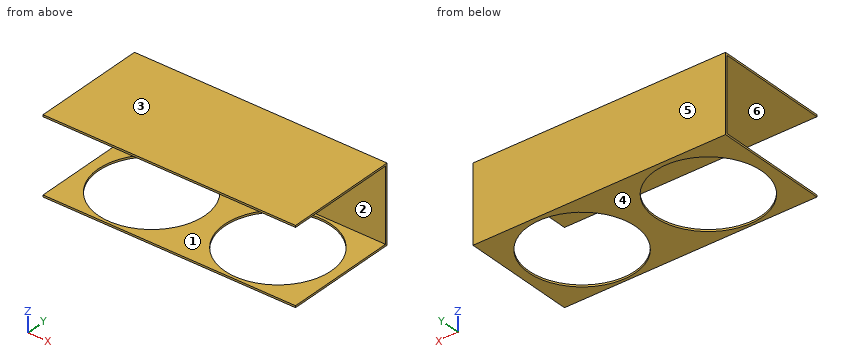
```python
from build123d import *

# Parameters (mm, degrees)
F0_W          = 270
F0_H          = 2
F0_H_2        = 120
F0_R          = 57
F1_DEPTH      = 2
F2_DEPTH      = 80
F3_W          = 270
F3_H          = 2
F4_DEPTH      = 120
F4_DEPTH_BACK = 2


with BuildPart() as f1:
    # F0 (on Top) → F1 (new body)
    with BuildSketch(Plane.XY):
        with Locations((13.665279, 62.509182)):
            Rectangle(F0_W, F0_H)
        with Locations((13.665279, 1.509182)):
            Rectangle(F0_W, F0_H_2)
        with Locations((-53.288383, 1.509182)):
            Circle(F0_R, mode=Mode.SUBTRACT)
        with Locations((81.711617, 1.509182)):
            Circle(F0_R, mode=Mode.SUBTRACT)
    extrude(amount=F1_DEPTH)

    # F0 (on Top) → F2 (join)
    with BuildSketch(Plane.XY):
        with Locations((13.665279, 62.509182)):
            Rectangle(F0_W, F0_H)
    extrude(amount=F2_DEPTH)

    # F3 (on face) → F4 (join, two sides)
    with BuildSketch(Plane.XZ.offset(-61.509182)) as f4_sk:
        with Locations((13.665279, 81)):
            Rectangle(F3_W, F3_H)
    extrude(amount=F4_DEPTH)
    extrude(f4_sk.sketch, amount=-F4_DEPTH_BACK)


solid = f1.part
```
Geometry check sheet. Reference: the model listing, model coordinates, mm. Face numbers are marked on the shaded views. A direction names the side the tool comes from. Coordinates: 2 decimals unless noted, no trailing zeros. Order: outer loops, then holes, each group sorted by start corner. A loop starts at its lowest first (then second) coordinate and runs counter-clockwise, first axis right, second up. Notation, with made-up numbers: (30, -32) - (59, -32) arc R20 ccw to (59, -6) - close; hole circle Ø1 at (6, -38.5). An arc over 180 degrees is marked (long way). Answer as a JSON object with one key per item and string values. Group by question number.
Item 1: Sectioned sample at B-B, the plane y = 22.5. Record the cut outline in (x, z), and give its area (3 significant figures).
Item 2: Sectioned sample at D-D, the plane z = 77. Record the cut outline in (x, y), and give its area (3 significant figures).
Item 3: Sectioned sample at C-C, the plane x = 13.5. Record the cut outline in (y, z), and give its area (3 significant figures).
Item 4: Tool access check on the marked faces 5 and 6. Record the directions out of +Z, -Z, +X, -X, +Y, -Y that give a thin tool (end or side, any length) a straight path to the whole face; none if there is none.
Item 5: Scan lines: probe 1 along Z at (x, y) = (20, -13); probe 2 along Y at (x, z) = (-15, 78); probe 3 along Z at (x, y) = (27, 5.5). Record each from-to range of solid material in increasing order.
Item 6: Depth check by flat-ended pin: pin 1 Ø1.5 at (x, y) = (-29, -27) entering from -Z; pin 2 Ø1 at (x, z) = (56, 50) entering from -Y. Enter the tip coordinate at first touch or a pass-through.
Item 7: Sectioned sample at A-A, the plane x = -37. Record the cut outline in (y, z).
Item 8: Draft check along Z on the marked faces 1, 2, 3 and 4. Enter one of: +Z half, -Z half, draft (parallel to the pull), parting line (faces both ways), or undercut.
Resolved:
{
 "1": {"outline": "(-121.33, 0) - (-106.28, 0) - (-106.28, 2) - (-121.33, 2) - close; (-121.33, 80) - (148.67, 80) - (148.67, 82) - (-121.33, 82) - close; (-0.29, 0) - (28.72, 0) - (28.72, 2) - (-0.29, 2) - close; (134.71, 0) - (148.67, 0) - (148.67, 2) - (134.71, 2) - close", "area": "656 mm^2"},
 "2": {"outline": "(-121.33, 61.51) - (148.67, 61.51) - (148.67, 63.51) - (-121.33, 63.51) - close", "area": "540 mm^2"},
 "3": {"outline": "(-58.49, 0) - (63.51, 0) - (63.51, 82) - (-58.49, 82) - (-58.49, 80) - (61.51, 80) - (61.51, 2) - (-58.49, 2) - close", "area": "644 mm^2"},
 "4": {"face 5": "+Z, -Z, +X, -X, +Y", "face 6": "+X, -X, -Y"},
 "5": {"probe 1": "0 to 2, 80 to 82", "probe 2": "61.51 to 63.51", "probe 3": "80 to 82"},
 "6": {"pin 1": "z = 80", "pin 2": "y = 61.51"},
 "7": {"outline": "(-58.49, 0) - (-53.11, 0) - (-53.11, 2) - (-58.49, 2) - close; (-58.49, 80) - (61.51, 80) - (61.51, 2) - (56.13, 2) - (56.13, 0) - (63.51, 0) - (63.51, 82) - (-58.49, 82) - close"},
 "8": {"face 1": "undercut", "face 2": "undercut", "face 3": "+Z half", "face 4": "-Z half"}
}
